Design review of the part built by this model. Coordinates are the model's own, in mm. Face numbers are marked on the shaded views. A direction names the side the tool comes from. Coordinates: 2 decimals unless noted, no trailing zeros. Write each loop counter-clockwise with the first axis right and the second up, starting at its lowest first coordinate (ties: lowest second). Pieces come first, ordered by that corner, then holes.
Q1. Machinability: for the marked faces 1, 2 and 3, which of the approach directions +Z, -Z, +X, -X, +Y, -Y give a long, thin tool a straight path to every point of the face, cutting with its end or side? Answer none if there is none.
Q2. Add section A-A, the plane z = 0. Give the boundary of the cut face in (x, y), plus the area to 3 significant figures.
Q3. Add section D-D, the plane y = 2. Give the boundary of the cut face in (x, z), plus the area to 3 significant figures.
Q4. Add section C-C, the plane y = 8. Give the boundary of the cut face in (x, z).
Q5. The part is to be moulded in two halves that separate along Z. For the marked faces 4, 5 and 6, say which applies: +Z half, -Z half, draft (parallel to the pull), parting line (faces both ways), or undercut.
Q6. To check wall thickness, follow probe 1 along Z at (x, y) = (-12, 12.45); probe 2 along X at (y, z) = (4.15, 0); probe 3 along X at (y, z) = (1.3, 0). State the ranges of each line that lie inside material, in increasing order.
Q7. Clearance check with flat-ended pins moving along their axes: pin 1 Ø2 at (x, z) = (-11.5, 28.5) entering from -Y; pin 2 Ø10 at (x, z) = (-4, 15) entering from +Y; pin 3 Ø4 at (x, z) = (-9, 1.5) entering from -Y; pin 4 Ø5.5 at (x, z) = (-12, -27.7) entering from -Y. State where each tip first meets the part, or that it passes through.
Q8. Add section B-B, the plane z = 27.7. Give the boundary of the cut face in (x, y).
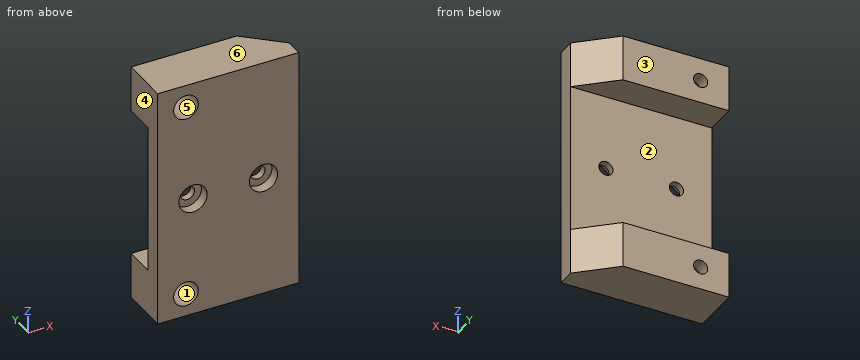
Autodesk Inventor part; units mm, degrees
ref_plane "YZ Plane" through (0, 0, 0) normal (1, 0, 0) x (0, 1, 0)
ref_plane "XZ Plane" through (0, 0, 0) normal (0, 1, 0) x (-1, 0, 0)
ref_plane "XY Plane" through (0, 0, 0) normal (0, 0, 1) x (1, 0, 0)
sketch "Skizze1" plane through (0, 0, 0) normal (0, 1, 0) x (-1, 0, 0)
  line L0 (-20, 34.2) -> (20, 34.2)
  line L1 (20, 34.2) -> (20, -34.2)
  line L2 (20, -34.2) -> (-20, -34.2)
  line L3 (-20, -34.2) -> (-20, 34.2)
  line L4 (-20, 34.2) -> (20, -34.2) construction
  line L5 (20, 34.2) -> (-20, -34.2) construction
  point P0 (0, 0)
  dimension "d0" = 40
  dimension "d1" = 68.4
extrude "Extrusion1" add sketch "Skizze1" along normal blind 5
sketch "Skizze5" plane through (0, 0, 0) normal (0, -1, 0) x (1, 0, 0)
  line L0 (20, 34.2) -> (-20, 34.2)
  line L1 (-20, 34.2) -> (-20, -34.2)
  line L2 (-20, -34.2) -> (20, -34.2)
  line L3 (20, -34.2) -> (20, 34.2)
  line L4 (32.3204, 0) -> (-38.6965, 0) construction
  point P0 (0, 0)
  point P1 (-10, 0)
  point P2 (10, 0)
  dimension "d32" = 10
  dimension "d33" = 20
hole "Bohrung3" at (-10, 0, 0) at (10, 0, 0) direction (0, 1, 0) diameter 4 end through all counterbore diameter 8 counterbore depth 3
sketch "Skizze6" plane through (0, 5, 0) normal (0, 1, 0) x (1, 0, 0)
  circle A0 centre (-10, 0) radius 2
  circle A1 centre (10, 0) radius 2
  line L0 (-20, -34.2) -> (20, -34.2)
  line L1 (20, -34.2) -> (20, 34.2)
  line L2 (20, 34.2) -> (-20, 34.2)
  line L3 (-20, 34.2) -> (-20, -34.2)
  line L4 (-20, 34.2) -> (10, 34.2)
  line L5 (10, 34.2) -> (10, 21.2)
  line L6 (10, 21.2) -> (-20, 21.2)
  line L7 (-20, 21.2) -> (-20, 34.2)
  line L8 (-35, 0) -> (35, 0)
  line L9 (-20, -34.2) -> (10, -34.2)
  line L10 (10, -34.2) -> (10, -21.2)
  line L11 (10, -21.2) -> (-20, -21.2)
  line L12 (-20, -21.2) -> (-20, -34.2)
  point P0 (0, 0)
  dimension "d41" = 30
  dimension "d42" = 13
extrude "Extrusion3" add sketch "Skizze6" along normal blind 9 contours L3 L2 L5 L6 | L11 L10 L0 L3
sketch "Skizze8" plane through (0, 0, 0) normal (0, -1, 0) x (1, 0, 0)
  line L0 (-20, 34.2) -> (10, 34.2)
  line L1 (10, 34.2) -> (10, 21.2)
  line L2 (10, 21.2) -> (-20, 21.2)
  line L3 (-20, 21.2) -> (-20, 34.2)
  line L4 (-20, -34.2) -> (-20, -21.2)
  line L5 (-20, -21.2) -> (10, -21.2)
  line L6 (10, -21.2) -> (10, -34.2)
  line L7 (10, -34.2) -> (-20, -34.2)
  line L8 (-20, 21.2) -> (-20, 34.2)
  line L9 (-20, 27.7) -> (10, 27.7)
  line L10 (-20, 34.2) -> (-20, -34.2)
  line L11 (10, -21.2) -> (10, -34.2)
  line L12 (10, -27.7) -> (-20, -27.7)
  point P0 (0, 0)
  point P1 (-12, 27.7)
  point P2 (-12, -27.7)
  dimension "d46" = 8
  dimension "d47" = 8
hole "Bohrung4" at (-12, 0, 27.7) at (-12, 0, -27.7) direction (0, 1, 0) diameter 4 end through all counterbore diameter 7 counterbore depth 10
sketch "Skizze9" plane through (20, 0, -34.2) normal (0, 0, -1) x (-1, 0, 0)
  line L0 (40, 0) -> (0, 0)
  line L1 (40, 0) -> (40, 14)
  line L2 (10, 14) -> (40, 14)
  line L3 (10, 5) -> (10, 14)
  line L4 (0, 5) -> (10, 5)
  line L5 (0, 0) -> (0, 5)
  line L6 (0, 5) -> (10, 5)
  line L7 (0, 5) -> (10, 14)
  point P0 (20, 0)
extrude "Extrusion4" add sketch "Skizze9" against normal up to surface (13 mm away) contours L7 L3 L4
sketch "Skizze11" plane through (-20, 0, 34.2) normal (0, 0, 1) x (1, 0, 0)
  line L0 (30, 5) -> (30, 14)
  line L1 (30, 5) -> (40, 5)
  line L2 (30, 14) -> (40, 5)
  line L3 (40, 0) -> (40, 5)
  line L4 (30, 14) -> (40, 5)
  point P0 (20, 0)
extrude "Extrusion5" add sketch "Skizze11" against normal up to surface (13 mm away)
properties part number "Backplate"
Here are the results:
1. face 1: -Y
1. face 2: +X, -X, +Y
1. face 3: +Z, -Z, +X, -X, +Y
2. outline: (-20, 0) - (-14, 0) - (-14, 3) - (-12, 3) - (-12, 5) - (-20, 5) - close; (-8, 3) - (-6, 3) - (-6, 0) - (6, 0) - (6, 3) - (8, 3) - (8, 5) - (-8, 5) - close; (12, 3) - (14, 3) - (14, 0) - (20, 0) - (20, 5) - (12, 5) - close
2. area: 136 mm2
3. outline: (-20, -34.2) - (20, -34.2) - (20, 34.2) - (-20, 34.2) - close; hole circle Ø7 at (-12, -27.7); hole circle Ø7 at (-12, 27.7); hole circle Ø8 at (-10, 0); hole circle Ø8 at (10, 0)
3. area: 2,560 mm2
4. outline: (-20, -34.2) - (16.67, -34.2) - (16.67, -21.2) - (-20, -21.2) - close; (-20, 21.2) - (16.67, 21.2) - (16.67, 34.2) - (-20, 34.2) - close; hole circle Ø7 at (-12, -27.7); hole circle Ø7 at (-12, 27.7)
5. face 4: draft
5. face 5: undercut
5. face 6: +Z half
6. probe 1: z = -34.2 to -29.7, -25.7 to -21.2, 21.2 to 25.7, 29.7 to 34.2
6. probe 2: x = -20 to -12, -8 to 8, 12 to 20
6. probe 3: x = -20 to -14, -6 to 6, 14 to 20
7. pin 1: passes through
7. pin 2: stops at y = 5
7. pin 3: stops at y = 3
7. pin 4: stops at y = 10
8. outline: (-20, 0) - (-15.5, 0) - (-15.5, 10) - (-14, 10) - (-14, 14) - (-20, 14) - close; (-10, 10) - (-8.5, 10) - (-8.5, 0) - (20, 0) - (20, 5) - (10, 14) - (-10, 14) - close
